The model under review builds one solid part; all positions refer to its coordinate system, in mm. Round coordinates to 2 decimals unless told otherwise and drop trailing zeros. Loops run counter-clockwise (first coordinate to the right, second up) from the corner with the lowest first, then second, coordinate; pieces in that order, holes last. Notation, with made-up numbers: M 69,20 L 98,20 A14 cw 98,25 Z; hole C 42.5,9 d10. An arc over 180 degrees is marked long. Answer in a Markdown table with one row per item. Add a question column.
from build123d import *

# Parameters (mm, degrees)
IZIM1_R                     = 35
IZIM1_R_2                   = 25
Y_KSEKLIK_EKSTR_ZYON1_DEPTH = 20
RADYUS1_R                   = 2


with BuildPart() as part:
    # Çizim1 → Yükseklik-Ekstrüzyon1 (new body)
    with BuildSketch(Plane.XY):
        Circle(IZIM1_R)
        Circle(IZIM1_R_2, mode=Mode.SUBTRACT)
    extrude(amount=Y_KSEKLIK_EKSTR_ZYON1_DEPTH)

    # Radyus1
    radyus1_edges = [part.edges().sort_by_distance(p)[0] for p in [
        (-35, 0, 0),
        (-35, 0, 20),
        (-25, 0, 0),
        (-25, 0, 20),
    ]]
    fillet(radyus1_edges, radius=RADYUS1_R)


solid = part.part
1. Take a section at A-A, the plane x = 0. State the section outline as (y, z) points, and give its area (3 significant figures).
2. To check wall thickness, follow probe 1 along Y at (x, z) = (0, 14.75); probe 2 along X at (y, z) = (0.5, 18) (3 decimals); probe 3 along X at (y, z) = (9, 8). State the ranges of each line that lie inside material, in increasing order.
3. Take a section at C-C, the plane z = 15.5. State the section outline as (x, y) points.
4. For pin 1 Ø2 at (y, z) = (15.5, 14) entering from +X; pin 2 Ø6 at (x, z) = (-17, 14.5) entering from +Y; pin 3 Ø2 at (x, z) = (-20, 7.5) entering from -Y, all flat-tipped, find the tip position at first contact; note any pin that passes through.
5. Mouldability with a two-part tool opening along Y and no side actions: class faces 1 (the cylindrical face through (23.846, 7.509, 9.888)), 2 (the cylindrical face through (-28, -21, 10)), 3 (the flat face through (-12.4, -24.3, 20)) as released by +Y, released by -Y, zero draft, split by the parting line, or undercut.
Check sheet entries:
| question | item | result |
|---|---|---|
| 1 | outline | M -35,2 A2 ccw -33,0 L -27,0 A2 ccw -25,2 L -25,18 A2 ccw -27,20 L -33,20 A2 ccw -35,18 Z; M 25,2 A2 ccw 27,0 L 33,0 A2 ccw 35,2 L 35,18 A2 ccw 33,20 L 27,20 A2 ccw 25,18 Z |
| 1 | area | 393 mm^2 |
| 2 | probe 1 | y = -35 to -25, 25 to 35 |
| 2 | probe 2 | x = -34.996 to -24.995, 24.995 to 34.996 |
| 2 | probe 3 | x = -33.82 to -23.32, 23.32 to 33.82 |
| 3 | outline | C 0,0 d70; hole C 0,0 d50 |
| 4 | pin 1 | stops at x = 31.86 |
| 4 | pin 2 | stops at y = 32.08 |
| 4 | pin 3 | stops at y = -29.39 |
| 5 | face 1 | undercut |
| 5 | face 2 | split by the parting line |
| 5 | face 3 | zero draft |
